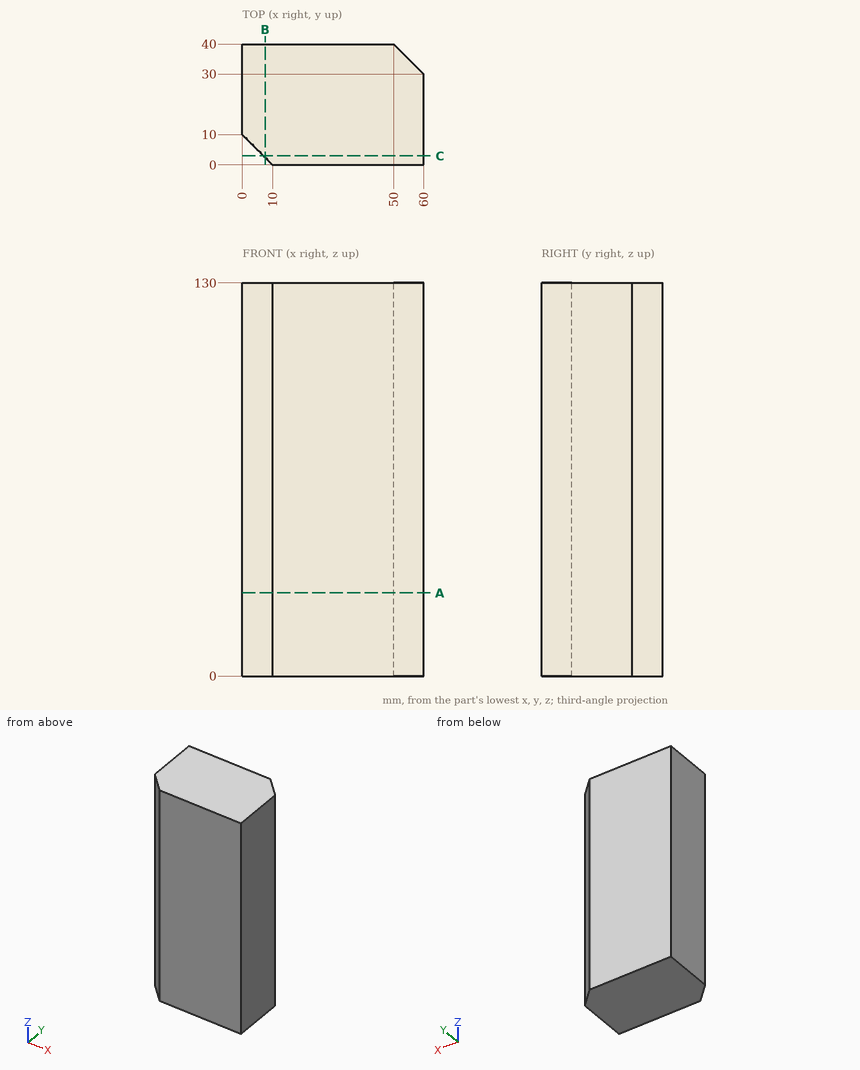
For this review, use the dimensioned drawing (mm, ordinates from the lowest corner) and the shaded views. Round coordinates to 2 decimals unless told otherwise and drop trailing zeros. Order: outer loops, then holes, each group sorted by start corner. A loop starts at its lowest first (then second) coordinate and runs counter-clockwise, first axis right, second up. Notation, with made-up numbers: (-16, 23.5) - (13, 23.5) arc R37 cw to (13, 61.5) - close; hole circle Ø1 at (85, 46.25). An arc over 180 degrees is marked (long way). Use one line per item in the form item = value.
Q1. Add section B-B on x = 7.5. Give the boundary of the cut face in (y, z).
Response values:
outline = (2.5, 0) - (40, 0) - (40, 130) - (2.5, 130) - close
Q2. Add section C-C on y = 3. Give the boundary of the cut face in (x, z).
Response values:
outline = (7, 0) - (60, 0) - (60, 130) - (7, 130) - close
Q3. Add section A-A on z = 27.5. Give the boundary of the cut face in (x, y).
Response values:
outline = (0, 10) - (10, 0) - (60, 0) - (60, 30) - (50, 40) - (0, 40) - close
Q4. To check wall thickness, follow line 1 (X direction, y = 9, z = 52.5); line 2 (Y direction, x = 52, z = 72.5); line 3 (X direction, y = 37, z = 35.5). State the ranges of each line that lie inside material, in increasing order.
Response values:
line_1 = 1 to 60
line_2 = 0 to 38
line_3 = 0 to 53
